Source: CAD feature listing. Evaluate the final solid. Frame: model axes, mm. A direction names the side the tool comes from. Round coordinates to 2 decimals unless told otherwise and drop trailing zeros. Order: outer loops, then holes, each group sorted by start corner. A loop starts at its lowest first (then second) coordinate and runs counter-clockwise, first axis right, second up. Notation, with made-up numbers: (81, 13.25) - (91, 13.25) arc R29 cw to (91, 33.25) - close; hole circle Ø7 at (42.5, 30). An arc over 180 degrees is marked (long way). Return JSON: item names as keys, results as strings. Group by question number.
1) Section A-A, the plane z = -60. Return loops of the section in (x, y), plus the area to 3 significant figures.
2) Section C-C, the plane y = 10.7. Return loops of the section in (x, z).
3) Section B-B, the plane x = 55. Return loops of the section in (y, z).
4) Mould query, pull axis X, two halves, no side actions, for faces 6 (the flat face through (-2.737, 12, -73)), 7 (the flat face through (-2, 11, -120)), 8 (the cylindrical face through (91.451, -0.986, -58.154)). Classes: pulls with the +X half, pulls with the -X half, needs draft (parallel to the pull), parting line crosses it, or undercut.
5) Ray query, line 1 (Y direction, x = 93, z = -73.5); line 2 (X direction, y = 6.25, z = -114.5); line 3 (Z direction, x = 102, y = 12.25). Return the intervals inside material, ascending. Write a range as from..to.
6) Section D-D, the plane x = 95. Return loops of the section in (y, z).
7) Access query for faces 1 (the flat face through (46, 0, -48)), 2 (the cylindrical face through (85.781, -0.986, -83.915)), 3 (the flat face through (-0.737, 12, -73)), 4 (the flat face through (46, -2, -48)), 5 (the flat face through (-2, 11, -25)). Directions: +Z, -Z, +X, -X, +Y, -Y. A direction counts if a zero-diameter tool reaches every point of the face in a straight line with its end or side. Return the directions, or none.
8) Contact query for flat-ended pins moving along their axis: P1, Ø4, axis at x = 64, z = -50, coming from the +Y side; P2, Ø1.4, axis at y = 15.5, z = 1, coming from the -X side; P3, Ø1.6, axis at x = 78.5, y = -1, coming from the -Z side; P4, Ø8, axis at x = 23.5, y = 19.5, coming from the +Z side. Output: stop coordinate, or through.
```python
from build123d import *

# Parameters (mm, degrees)
BRIDA_BASE1_DEPTH               = 2
BRIDA_DE_ARISTA1_DEPTH          = 95
BRIDA_DE_ARISTA2_DEPTH          = 95
CROQUIS16_R                     = 4
CORTAR_EXTRUIR3_DEPTH           = 10
CROQUIS17_R                     = 8.95
CORTAR_EXTRUIR5_DEPTH           = 2
CORTAR_EXTRUIR5_DRAFT           = -45
CORTAR_EXTRUIR5_PROFILE_2_DEPTH = 2
CORTAR_EXTRUIR5_PROFILE_2_DRAFT = -45
CROQUIS18_R                     = 8.95
CORTAR_EXTRUIR6_DEPTH           = 2
CORTAR_EXTRUIR6_DRAFT           = -45
CORTAR_EXTRUIR6_PROFILE_2_DEPTH = 2
CORTAR_EXTRUIR6_PROFILE_2_DRAFT = -45


# Sheet-metal steps are written as plain solids
with BuildPart() as part:
    # Croquis1 → Brida base1 (new body)
    with BuildSketch(Plane(origin=(0, 0, 0), x_dir=(1, 0, 0), z_dir=(0, 1, 0))):
        with BuildLine():
            Line((0, 25), (25, 0))
            Line((25, 0), (120, 0))
            ThreePointArc((120, 0), (84.852813742, 84.852813742), (0, 120))
            Line((0, 120), (0, 25))
        make_face()
    extrude(amount=-BRIDA_BASE1_DEPTH)

    # Brida de arista1 section (across the edge) → Brida de arista1 (add)
    with BuildSketch(Plane(origin=(25, 0, 0.7366), x_dir=(0, 0, -1), z_dir=(1, 0, 0))):
        with BuildLine():
            Line((-2, 0.7366), (-2, 23.4))
            Line((-2, 23.4), (0, 23.4))
            Line((0, 23.4), (0, 0.7366))
            ThreePointArc((0, 0.7366), (0.215745145, 0.215745145), (0.7366, 0))
            Line((0.7366, 0), (0.7366, -2))
            ThreePointArc((0.7366, -2), (-1.198468417, -1.198468417), (-2, 0.7366))
        make_face()
    extrude(amount=BRIDA_DE_ARISTA1_DEPTH)

    # Brida de arista2 section (across the edge) → Brida de arista2 (add)
    with BuildSketch(Plane(origin=(-0.7366, 0, -120), x_dir=(1, 0, 0), z_dir=(0, 0, 1))):
        with BuildLine():
            Line((-2, 0.7366), (-2, 23.4))
            Line((-2, 23.4), (0, 23.4))
            Line((0, 23.4), (0, 0.7366))
            ThreePointArc((0, 0.7366), (0.215745145, 0.215745145), (0.7366, 0))
            Line((0.7366, 0), (0.7366, -2))
            ThreePointArc((0.7366, -2), (-1.198468417, -1.198468417), (-2, 0.7366))
        make_face()
    extrude(amount=BRIDA_DE_ARISTA2_DEPTH)

    # Croquis16 → Cortar-Extruir3 (cut)
    with BuildSketch(Plane(origin=(0, 0, 0), x_dir=(1, 0, 0), z_dir=(0, 1, 0))):
        with Locations(Location((55, 60, 0), (0, 0, 270))):
            Circle(CROQUIS16_R)
        with Locations(Location((95, 60, 0), (0, 0, 270))):
            Circle(CROQUIS16_R)
        Polygon((70, 40), (72.5, 40), (72.5, 80), (77.5, 80), (77.5, 40), (80, 40), (80, 85), (70, 85), align=None)
    extrude(amount=-CORTAR_EXTRUIR3_DEPTH, mode=Mode.SUBTRACT)


with BuildPart() as cortar_extruir5_tool:
    # Croquis17 → Cortar-Extruir5 (with draft: the straight prism first)
    with BuildSketch(Plane(origin=(0, 0, 0.7366), x_dir=(-1, 0, 0), z_dir=(0, 0, -1))):
        with Locations((-42.2634, 10.7)):
            Circle(CROQUIS17_R)
    extrude(amount=-CORTAR_EXTRUIR5_DEPTH)
    # Cortar-Extruir5: the draft: its side faces are tilted about the plane it starts from
    cortar_extruir5_sides = [cortar_extruir5_tool.faces().sort_by_distance(p)[0] for p in [
        (51.2134, 10.7, 1.7366),
    ]]
    draft(cortar_extruir5_sides, Plane(origin=(0, 0, 0.7366), x_dir=(-1, 0, 0), z_dir=(0, 0, -1)), CORTAR_EXTRUIR5_DRAFT)


with BuildPart() as part_1:
    add(part.part)

    # Cortar-Extruir5: cut by cortar_extruir5_tool
    add(cortar_extruir5_tool.part, mode=Mode.SUBTRACT)


with BuildPart() as cortar_extruir5_profile_2_tool:
    # Croquis17 → Cortar-Extruir5 profile 2 (with draft: the straight prism first)
    with BuildSketch(Plane(origin=(0, 0, 0.7366), x_dir=(-1, 0, 0), z_dir=(0, 0, -1))):
        with Locations((-82.2634, 10.7)):
            Circle(CROQUIS17_R)
    extrude(amount=-CORTAR_EXTRUIR5_PROFILE_2_DEPTH)
    # Cortar-Extruir5 profile 2: the draft: its side faces are tilted about the plane it starts from
    cortar_extruir5_profile_2_sides = [cortar_extruir5_profile_2_tool.faces().sort_by_distance(p)[0] for p in [
        (91.2134, 10.7, 1.7366),
    ]]
    draft(cortar_extruir5_profile_2_sides, Plane(origin=(0, 0, 0.7366), x_dir=(-1, 0, 0), z_dir=(0, 0, -1)), CORTAR_EXTRUIR5_PROFILE_2_DRAFT)


with BuildPart() as part_2:
    add(part_1.part)

    # Cortar-Extruir5 profile 2: cut by cortar_extruir5_profile_2_tool
    add(cortar_extruir5_profile_2_tool.part, mode=Mode.SUBTRACT)


with BuildPart() as cortar_extruir6_tool:
    # Croquis18 → Cortar-Extruir6 (with draft: the straight prism first)
    with BuildSketch(Plane(origin=(-0.7366, 0, 0), x_dir=(0, 0, -1), z_dir=(1, 0, 0))):
        with Locations((42.2634, 10.7)):
            Circle(CROQUIS18_R)
    extrude(amount=-CORTAR_EXTRUIR6_DEPTH)
    # Cortar-Extruir6: the draft: its side faces are tilted about the plane it starts from
    cortar_extruir6_sides = [cortar_extruir6_tool.faces().sort_by_distance(p)[0] for p in [
        (-1.7366, 10.7, -33.3134),
    ]]
    draft(cortar_extruir6_sides, Plane(origin=(-0.7366, 0, 0), x_dir=(0, 0, -1), z_dir=(1, 0, 0)), CORTAR_EXTRUIR6_DRAFT)


with BuildPart() as part_3:
    add(part_2.part)

    # Cortar-Extruir6: cut by cortar_extruir6_tool
    add(cortar_extruir6_tool.part, mode=Mode.SUBTRACT)


with BuildPart() as cortar_extruir6_profile_2_tool:
    # Croquis18 → Cortar-Extruir6 profile 2 (with draft: the straight prism first)
    with BuildSketch(Plane(origin=(-0.7366, 0, 0), x_dir=(0, 0, -1), z_dir=(1, 0, 0))):
        with Locations((82.2634, 10.7)):
            Circle(CROQUIS18_R)
    extrude(amount=-CORTAR_EXTRUIR6_PROFILE_2_DEPTH)
    # Cortar-Extruir6 profile 2: the draft: its side faces are tilted about the plane it starts from
    cortar_extruir6_profile_2_sides = [cortar_extruir6_profile_2_tool.faces().sort_by_distance(p)[0] for p in [
        (-1.7366, 10.7, -73.3134),
    ]]
    draft(cortar_extruir6_profile_2_sides, Plane(origin=(-0.7366, 0, 0), x_dir=(0, 0, -1), z_dir=(1, 0, 0)), CORTAR_EXTRUIR6_PROFILE_2_DRAFT)


with BuildPart() as part_4:
    add(part_3.part)

    # Cortar-Extruir6 profile 2: cut by cortar_extruir6_profile_2_tool
    add(cortar_extruir6_profile_2_tool.part, mode=Mode.SUBTRACT)


solid = part_4.part
```
Geometry check:
{
 "1": {"outline": "(-2.74, 0.74) arc R2.74 ccw to (0, -2) - (51, -2) - (51, 0) - (0, 0) arc R0.74 cw to (-0.74, 0.74) - (-0.74, 23.4) - (-2.74, 23.4) - close; (59, -2) - (70, -2) - (70, 0) - (59, 0) - close; (72.5, -2) - (77.5, -2) - (77.5, 0) - (72.5, 0) - close; (80, -2) - (91, -2) - (91, 0) - (80, 0) - close; (99, -2) - (103.92, -2) - (103.92, 0) - (99, 0) - close", "area": "217 mm2"},
 "2": {"outline": "(-2.74, -120) - (-0.74, -120) - (-0.74, -91.21) - (-2.74, -89.21) - close; (-2.74, -75.31) - (-0.74, -73.31) - (-0.74, -51.21) - (-2.74, -49.21) - close; (-2.74, -35.31) - (-0.74, -33.31) - (-0.74, -25) - (-2.74, -25) - close; (25, 0.74) - (33.31, 0.74) - (35.31, 2.74) - (25, 2.74) - close; (49.21, 2.74) - (51.21, 0.74) - (73.31, 0.74) - (75.31, 2.74) - close; (89.21, 2.74) - (91.21, 0.74) - (120, 0.74) - (120, 2.74) - close"},
 "3": {"outline": "(-2, -106.65) - (0, -106.65) - (0, -64) - (-2, -64) - close; (-2, -56) - (0, -56) - (0, 0) arc R0.74 cw to (0.74, 0.74) - (23.4, 0.74) - (23.4, 2.74) - (0.74, 2.74) arc R2.74 ccw to (-2, 0) - close"},
 "4": {"face 6": "pulls with the -X half", "face 7": "needs draft", "face 8": "undercut"},
 "5": {"line 1": "-2..0", "line 2": "-2.74..-0.74", "line 3": "0.74..2.74"},
 "6": {"outline": "(-2, -73.31) - (0, -73.31) - (0, -64) - (-2, -64) - close; (-2, -56) - (0, -56) - (0, 0) arc R0.74 cw to (0.74, 0.74) - (23.4, 0.74) - (23.4, 2.74) - (0.74, 2.74) arc R2.74 ccw to (-2, 0) - close"},
 "7": {"face 1": "-Z, +X, +Y", "face 2": "-Z, +X, +Y, -Y", "face 3": "+Z, -Z, +X, +Y", "face 4": "+Z, -Z, +X, -X, -Y", "face 5": "+Z, -X, +Y, -Y"},
 "8": {"P1": "y = 0", "P2": "x = 25", "P3": "z = -91.45", "P4": "z = 2.74"}
}
